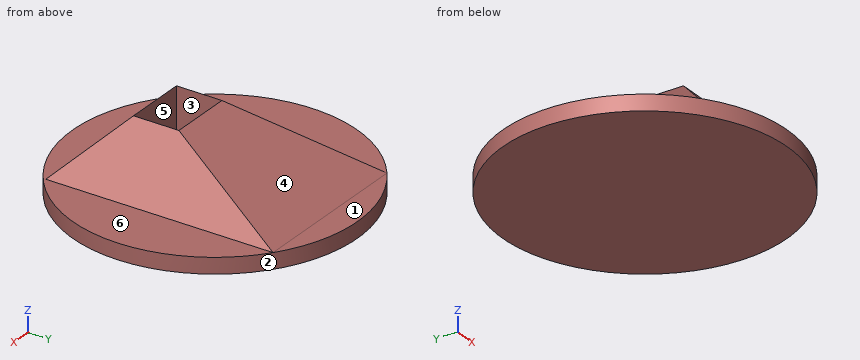
Autodesk Inventor part; units mm, degrees
ref_plane "Arbeitsebene3" through (0, 0, 0.5) normal (0, 0, 1) x (1, 0, 0)
ref_plane "YZ Plane" through (0, 0, 0) normal (1, 0, 0) x (0, 1, 0)
ref_plane "XZ Plane" through (0, 0, 0) normal (0, 1, 0) x (-1, 0, 0)
sketch "Skizze1" plane through (0, 0, 0) normal (0, 0, 1) x (1, 0, 0)
  circle A0 centre (0, 0) radius 9
  dimension "d0" = 18
extrude "Extrusion1" add sketch "Skizze1" along normal mid plane 1
sketch "Skizze2" plane through (0, 0, 0.5) normal (0, 0, 1) x (1, 0, 0)
  line L0 (-5.3, -0.925) -> (-2, -0.925)
  line L1 (-2, -0.925) -> (-2, -3.8)
  line L2 (-2, -3.8) -> (2, -3.8)
  line L3 (2, -3.8) -> (2, -0.925)
  line L4 (2, -0.925) -> (5.3, -0.925)
  line L5 (5.3, -0.925) -> (5.3, -7.1)
  line L6 (5.3, -7.1) -> (-5.3, -7.1)
  line L7 (-5.3, -7.1) -> (-5.3, -0.925)
  point P0 (0, 0)
  point P1 (0, -3.8)
  dimension "d3" = 4
  dimension "d4" = 2.875
  dimension "d5" = 3.3
  dimension "d6" = 3.3
  dimension "d17" = 3.8
extrude "Extrusion3" add sketch "Skizze2" along normal blind 3.3
ref_plane "Arbeitsebene3" through (0, 0, 0.5) normal (0, 0, 1) x (1, 0, 0)
sketch "Skizze5" plane through (0, 0, 0.5) normal (0, 0, 1) x (1, 0, 0)
  line L0 (-2, -0.925) -> (-2, -3.8) construction
  line L1 (-2, -3.8) -> (2, -3.8) construction
  line L2 (2, -3.8) -> (2, -0.925) construction
  line L3 (2, -0.925) -> (5.3, -0.925) construction
  line L4 (5.3, -0.925) -> (5.3, -7.1) construction
  line L5 (5.3, -7.1) -> (-5.3, -7.1) construction
  line L6 (-5.3, -7.1) -> (-5.3, -0.925) construction
  line L7 (-5.3, -0.925) -> (-2, -0.925) construction
  circle A0 centre (0, 0) radius 9 construction
  line L8 (-5.3, -0.925) -> (-5.3, 7.2739)
  line L9 (-5.3, 7.2739) -> (5.3, 7.2739)
  circle A1 centre (0, 0) radius 9
  line L10 (5.3, 7.2739) -> (5.3, -0.925)
  line L11 (-5.3, -0.925) -> (5.3, -0.925)
  dimension "d26" = 8.1989
extrude "Extrusion4" add sketch "Skizze5" along normal up to surface (3.3 mm away) contours L8 L9 L10 L11
chamfer "Fase1" distance 3.3 angle 45 3 edges at (0, -7.1, 3.8) (5.3, 0.087, 3.8) (-5.3, 0.087, 3.8)
chamfer "Fase2" distance 3.3 distance2 8.1989 1 edges at (0, 7.2739, 3.8) measured on face at (0.6667, 7.2739, 1.6)
equation "\"d6\" = d5"
equation "\"d28\" = d26"
properties part number "Membran_Platte" material "Stahl"
CAD build for the part. Positions are in the model's coordinates, mm. Face numbers are marked on the shaded views. A direction names the side the tool comes from. Round coordinates to 2 decimals unless told otherwise and drop trailing zeros. Write each loop counter-clockwise with the first axis right and the second up, starting at its lowest first coordinate (ties: lowest second). Pieces come first, ordered by that corner, then holes. Notation, with made-up numbers: (22, 32) -> (50, 32) arc R10 ccw to (50, 49) -> close; hole circle Ø7 at (-33, 8.5). An arc over 180 degrees is marked (long way). Answer in a Markdown table with one row per item. Add a question column.
Item 1: Which spindle directions (+Z, -Z, +X, -X, +Y, -Y) get a long thin tool onto all of the face, cutting with end or side? Do the marked faces 1 and 2. Say none if no direction does.
Item 2: Mould opens along Y. For the marked faces 3, 4, 5 and 6 say: pulls with the +Y half, pulls with the -Y half, needs draft (parallel to the pull), parting line crosses it, or undercut.
Item 3: Saw through at D-D, the plane z = 0.25. Write the cut outline in (x, y), then the cut area to 3 significant figures.
Item 4: Drop flat-ended pins along their axis: pin 1 Ø1.4 at (x, y) = (-1.5, 8) entering from +Z; pin 2 Ø1.6 at (x, z) = (-1, 2) entering from +Y; pin 3 Ø2 at (x, z) = (2, 3.5) entering from -Y. Give the stop position or say it passes through.
Item 5: Drill centre lines: line 1 (Z direction, x = -7.5, y = -1.75); line 2 (Y direction, x = 1.5, z = 3.5) (3 decimals); line 3 (Y direction, x = -0.25, z = 2.5) (3 decimals). Where is each one in solid material? Low to high. Write a range as from..to.
Item 6: Saw through at B-B, the plane z = 2.85. Write the cut outline in (x, y) (3 decimals), then the cut area to 3 significant figures.
Findings below:
| question | item | result |
|---|---|---|
| 1 | face 1 | +Z, +X, -X, +Y |
| 1 | face 2 | +Z, -Z |
| 2 | face 3 | undercut |
| 2 | face 4 | pulls with the +Y half |
| 2 | face 5 | undercut |
| 2 | face 6 | needs draft |
| 3 | outline | circle Ø18 at (0, 0) |
| 3 | area | 254 mm^2 |
| 4 | pin 1 | stops at z = 0.5 |
| 4 | pin 2 | stops at y = 5.53 |
| 4 | pin 3 | stops at y = -5.1 |
| 5 | line 1 | z = -0.5..0.5 |
| 5 | line 2 | y = -4.1..-3.8, -0.925..-0.18 |
| 5 | line 3 | y = -5.1..-3.8, -0.925..2.305 |
| 6 | outline | (-2.95, -4.75) -> (2.95, -4.75) -> (2.95, 1.435) -> (-2.95, 1.435) -> close; hole (-2, -3.8) -> (2, -3.8) -> (2, -0.925) -> (-2, -0.925) -> close |
| 6 | area | 25.0 mm^2 |
